Answer from the drawing. Dimensions are ordinates in mm from the lowest x, y and z of the part. Coordinates: 2 decimals unless noted, no trailing zeros. Loops run counter-clockwise (first coordinate to the right, second up) from the corner with the lowest first, then second, coordinate; pieces in that order, holes last. Notation, with made-up numbers: (-24.5, 48) - (-13.5, 48) arc R17 cw to (-13.5, 74) - close; hole circle Ø9 at (24, 14.25). An arc over 180 degrees is marked (long way). Write each question's results on one line, items separated by ' | '. Start each with the question number.
1. A cutting plane is placed at C-C on z = 2. Determine the outline of the cut face in (x, y) (3 decimals), then the cut area to 3 significant figures.
2. A cutting plane is placed at D-D on x = 34.29. Determine the outline of the cut face in (y, z) (3 decimals).
3. A cutting plane is placed at A-A on x = 22.86. Determine the outline of the cut face in (y, z) (3 decimals).
4. Find the intervals of material crossed by line 1 along X through (y, z) = (16, 1.1); line 2 along X through (y, z) = (8.5, 1.75); line 3 along Y through (x, z) = (34.29, 1.7), in increasing order. Write a range as [from, to].
5. Each of these flat-tipped pins is pushed along its axis until it touches: P1, Ø1.5, axis at x = 8, z = 1.5, coming from the -Y side; P2, Ø1, axis at x = 51, z = 2.5, coming from the -Y side (3 decimals); P3, Ø4, axis at x = 11.43, y = 8.763, coming from the +Z side; P4, Ø1, axis at x = 49.5, z = 2, coming from the +Y side. Where does it stop, or does it pass through?
6. A cutting plane is placed at B-B on y = 1.5. Determine the outline of the cut face in (x, z) (3 decimals), then the cut area to 3 significant figures.
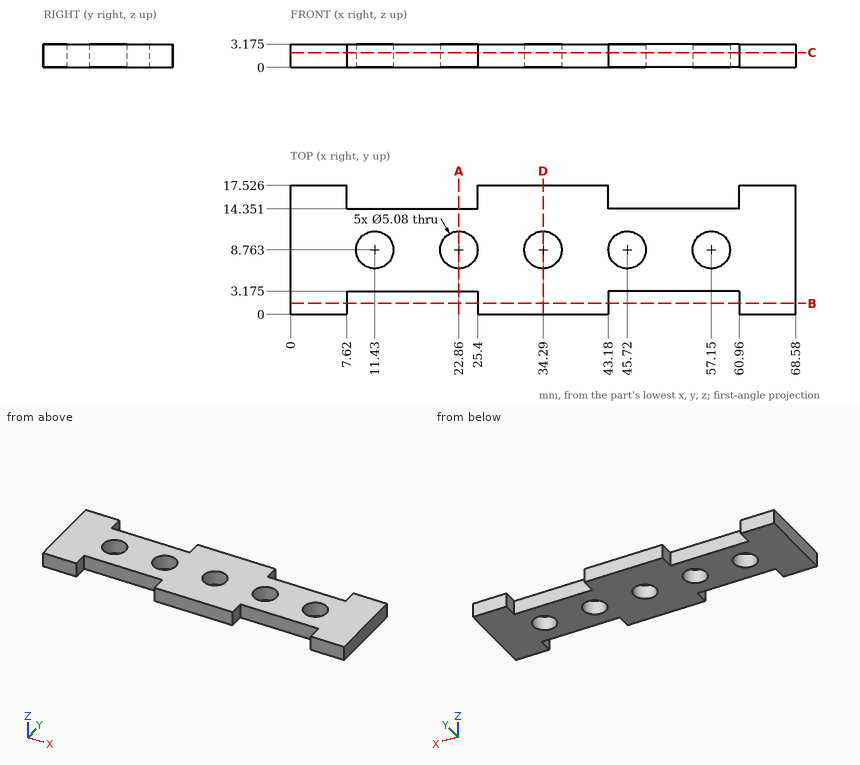
Values:
1) outline: (0, 0) - (7.62, 0) - (7.62, 3.175) - (25.4, 3.175) - (25.4, 0) - (43.18, 0) - (43.18, 3.175) - (60.96, 3.175) - (60.96, 0) - (68.58, 0) - (68.58, 17.526) - (60.96, 17.526) - (60.96, 14.351) - (43.18, 14.351) - (43.18, 17.526) - (25.4, 17.526) - (25.4, 14.351) - (7.62, 14.351) - (7.62, 17.526) - (0, 17.526) - close; hole circle Ø5.08 at (11.43, 8.763); hole circle Ø5.08 at (22.86, 8.763); hole circle Ø5.08 at (34.29, 8.763); hole circle Ø5.08 at (45.72, 8.763); hole circle Ø5.08 at (57.15, 8.763) | area: 875 mm^2
2) outline: (0, 0) - (6.223, 0) - (6.223, 3.175) - (0, 3.175) - close; (11.303, 0) - (17.526, 0) - (17.526, 3.175) - (11.303, 3.175) - close
3) outline: (3.175, 0) - (6.223, 0) - (6.223, 3.175) - (3.175, 3.175) - close; (11.303, 0) - (14.351, 0) - (14.351, 3.175) - (11.303, 3.175) - close
4) line 1: [0, 7.62], [25.4, 43.18], [60.96, 68.58] | line 2: [0, 8.9], [13.96, 20.33], [25.39, 31.76], [36.82, 43.19], [48.25, 54.62], [59.68, 68.58] | line 3: [0, 6.22], [11.3, 17.53]
5) P1: y = 0 | P2: y = 3.175 | P3: through | P4: y = 14.35
6) outline: (0, 0) - (7.62, 0) - (7.62, 3.175) - (0, 3.175) - close; (25.4, 0) - (43.18, 0) - (43.18, 3.175) - (25.4, 3.175) - close; (60.96, 0) - (68.58, 0) - (68.58, 3.175) - (60.96, 3.175) - close | area: 105 mm^2
